Model file for the job. Use its own axes, mm. A direction names the side the tool comes from. Coordinates: 2 decimals unless noted, no trailing zeros. Write each loop counter-clockwise with the first axis right and the second up, starting at its lowest first coordinate (ties: lowest second). Pieces come first, ordered by that corner, then holes. Notation, with made-up numbers: M -29,-5.5 L 18,-5.5 A25 cw 18,21.5 Z; hole C 89.5,70 d10. An arc over 180 degrees is marked long. One line per question, with ' | ' between items. Start each with the question number.
(1) Wall check: probe 1 along X at (y, z) = (1.15, 15.5) (3 decimals); probe 2 along X at (y, z) = (0.9, -23.57) (3 decimals); probe 3 along Z at (x, y) = (15, 3.25) (1 decimal). Give the ranges that are in metal, low to high.
(2) Flat gauge pins, fed straight in: pin 1 Ø17.5 at (x, z) = (-14, 19.5) entering from -Y; pin 2 Ø4.5 at (x, z) = (-15.5, 15.5) entering from -Y; pin 3 Ø2 at (x, y) = (-20.5, -1.5) entering from -Z; pin 4 Ø8 at (x, z) = (5.5, 3) entering from -Y. Where does each tip first touch, or does it go through?
(3) Tool access for faces 1 (the face through (-18, 0, -21)), 2 (the face through (-18, 2, 12.5)), 3 (the face through (-28.625, 2, 19)): list every direction of +Z, -Z, +X, -X, +Y, -Y with a clear straight run to the whole face (end or side of a thin tool).
(4) Cut at D-D (y = -1.75). Write the cut outline in (x, z) (3 decimals).
(5) Two-plate mould, pull along X, no slides. Class faces 4 (the face through (-6.625, 2, 0)), 5 (the face through (0, 4, -13)), 6 (the face through (-1.1, -2.75, -0.4)), 7 (the face through (25.68, 1.97, -22.23)): +X half, -X half, draft (parallel to the pull), parting line (faces both ways), or undercut.
(6) Cut at B-B (y = 1.75). Count the separate pieces of the cut face and the enclosed holes in it, plus the area to 3 significant figures.
(7) Cut at C-C (z = 23.57). Write the cut outline in (x, y) (3 decimals).
(8) Cut at A-A (z = 15.5). Write the cut outline in (x, y) (3 decimals), plus the area to 3 significant figures.
from build123d import *

# Parameters (mm, degrees)
SKETCH1_R              = 2
SKETCH1_R_2            = 2.5
BOSS_EXTRUDE1_DEPTH    = 4
CUT_EXTRUDE2_DEPTH     = 23
CHAMFER2_SIZE          = 1
CUT_EXTRUDE3_START     = -4
CUT_EXTRUDE3_OUTLINE_W = 22
CUT_EXTRUDE3_OUTLINE_H = 25
CUT_EXTRUDE3_DEPTH     = 4
BOSS_EXTRUDE2_REACH    = 66.132


# Read off the part's stored shape, not the designer's step: Cut-Extrude3
with BuildPart() as part:
    # Sketch1 → Boss-Extrude1 (new body)
    with BuildSketch(Plane(origin=(0, 0, 0), x_dir=(1, 0, 0), z_dir=(0, 1, 0))):
        with BuildLine():
            Line((25.625, 28.625), (-25.625, 28.625))
            ThreePointArc((-25.625, 28.625), (-27.746320344, 27.746320344), (-28.625, 25.625))
            Line((-28.625, 25.625), (-28.625, -25.625))
            ThreePointArc((-28.625, -25.625), (-27.746320344, -27.746320344), (-25.625, -28.625))
            Line((-25.625, -28.625), (25.625, -28.625))
            ThreePointArc((25.625, -28.625), (27.746320344, -27.746320344), (28.625, -25.625))
            Line((28.625, -25.625), (28.625, 25.625))
            ThreePointArc((28.625, 25.625), (27.746320344, 27.746320344), (25.625, 28.625))
        make_face()
        with Locations(Location((-15.5, 15.5, 0), (0, 0, 270))):
            Circle(SKETCH1_R, mode=Mode.SUBTRACT)
        with Locations(Location((-23.57, 23.57, 0), (0, 0, 270))):
            Circle(SKETCH1_R_2, mode=Mode.SUBTRACT)
        with Locations(Location((23.57, 23.57, 0), (0, 0, 270))):
            Circle(SKETCH1_R_2, mode=Mode.SUBTRACT)
        with Locations(Location((15.5, 15.5, 0), (0, 0, 270))):
            Circle(SKETCH1_R, mode=Mode.SUBTRACT)
        with Locations(Location((15.5, -15.5, 0), (0, 0, 270))):
            Circle(SKETCH1_R, mode=Mode.SUBTRACT)
        with Locations(Location((-15.5, -15.5, 0), (0, 0, 270))):
            Circle(SKETCH1_R, mode=Mode.SUBTRACT)
        with Locations(Location((-23.57, -23.57, 0), (0, 0, 270))):
            Circle(SKETCH1_R_2, mode=Mode.SUBTRACT)
        with Locations(Location((23.57, -23.57, 0), (0, 0, 270))):
            Circle(SKETCH1_R_2, mode=Mode.SUBTRACT)
    extrude(amount=BOSS_EXTRUDE1_DEPTH)

    # Sketch3 → Cut-Extrude2 (cut)
    with BuildSketch(Plane.XY.offset(11.5)):
        Polygon((-28.125, 4), (-27.125, 3), (-26.125, 4), align=None)
        Polygon((-25.125, 4), (-24.125, 3), (-23.125, 4), align=None)
        Polygon((-22.125, 4), (-21.125, 3), (-20.125, 4), align=None)
        Polygon((-19.125, 4), (-18.125, 3), (-17.125, 4), align=None)
        Polygon((-16.125, 4), (-15.125, 3), (-14.125, 4), align=None)
        Polygon((-13.125, 4), (-12.125, 3), (-11.125, 4), align=None)
        Polygon((-10.125, 4), (-9.125, 3), (-8.125, 4), align=None)
        Polygon((-7.125, 4), (-6.125, 3), (-5.125, 4), align=None)
        Polygon((-4.125, 4), (-3.125, 3), (-2.125, 4), align=None)
        Polygon((-1.125, 4), (-0.125, 3), (0.875, 4), align=None)
        Polygon((1.875, 4), (2.875, 3), (3.875, 4), align=None)
        Polygon((4.875, 4), (5.875, 3), (6.875, 4), align=None)
        Polygon((7.875, 4), (8.875, 3), (9.875, 4), align=None)
        Polygon((10.875, 4), (11.875, 3), (12.875, 4), align=None)
        Polygon((13.875, 4), (14.875, 3), (15.875, 4), align=None)
        Polygon((16.875, 4), (17.875, 3), (18.875, 4), align=None)
        Polygon((19.875, 4), (20.875, 3), (21.875, 4), align=None)
        Polygon((22.875, 4), (23.875, 3), (24.875, 4), align=None)
        Polygon((25.875, 4), (26.875, 3), (27.875, 4), align=None)
    extrude(amount=-CUT_EXTRUDE2_DEPTH, mode=Mode.SUBTRACT)

    # Chamfer2
    chamfer2_edges = [part.edges().sort_by_distance(p)[0] for p in [
        (26.875, 4, -11.5),
        (23.875, 4, -11.5),
        (20.875, 4, -11.5),
        (17.875, 4, -11.5),
        (14.875, 4, -11.5),
        (11.875, 4, -11.5),
        (8.875, 4, -11.5),
        (5.875, 4, -11.5),
        (2.875, 4, -11.5),
        (-0.125, 4, -11.5),
        (-3.125, 4, -11.5),
        (-6.125, 4, -11.5),
        (-9.125, 4, -11.5),
        (-12.125, 4, -11.5),
        (-15.125, 4, -11.5),
        (-18.125, 4, -11.5),
        (-21.125, 4, -11.5),
        (-24.125, 4, -11.5),
        (-27.125, 4, -11.5),
        (26.875, 4, 11.5),
        (23.875, 4, 11.5),
        (20.875, 4, 11.5),
        (17.875, 4, 11.5),
        (14.875, 4, 11.5),
        (11.875, 4, 11.5),
        (8.875, 4, 11.5),
        (5.875, 4, 11.5),
        (2.875, 4, 11.5),
        (-0.125, 4, 11.5),
        (-3.125, 4, 11.5),
        (-6.125, 4, 11.5),
        (-9.125, 4, 11.5),
        (-12.125, 4, 11.5),
        (-15.125, 4, 11.5),
        (-18.125, 4, 11.5),
        (-21.125, 4, 11.5),
        (-24.125, 4, 11.5),
        (-27.125, 4, 11.5),
    ]]
    chamfer(chamfer2_edges, length=CHAMFER2_SIZE - 0.0001)  # a hair under: the kernel refuses the full size

    # Cut-Extrude3 outline → Cut-Extrude3 (cut)
    with BuildSketch(Plane.XZ.offset(CUT_EXTRUDE3_START)):
        with Locations((-17.625, 0)):
            Rectangle(CUT_EXTRUDE3_OUTLINE_W, CUT_EXTRUDE3_OUTLINE_H)
    extrude(amount=CUT_EXTRUDE3_DEPTH, mode=Mode.SUBTRACT)

    # Boss-Extrude2: up to this face of the body (flat: up to its plane)
    boss_extrude2_end = Plane(part.part.faces().sort_by_distance((0, 2, 28.625))[0])
    # Sketch5 → Boss-Extrude2 (add, up to the picked face)
    with BuildSketch(Plane(origin=(0, 0, -28.625), x_dir=(-1, 0, 0), z_dir=(0, 0, -1)), mode=Mode.PRIVATE) as boss_extrude2_sk1:
        with BuildLine():
            Line((6.625, 0), (-4.249281585, 0))
            ThreePointArc((-4.249281585, 0), (1.187859207, -2.75), (6.625, 0))
        make_face()
    boss_extrude2_tool1 = split(extrude(boss_extrude2_sk1.sketch, amount=-BOSS_EXTRUDE2_REACH, mode=Mode.PRIVATE), bisect_by=boss_extrude2_end, keep=Keep.BOTH, mode=Mode.PRIVATE)
    add(boss_extrude2_tool1.solids().sort_by(Axis((-1.187859, -1.121798, -28.625), (0, 0, 1)))[0])


solid = part.part
Filled in:
1) probe 1: -28.625 to -17.5, -13.5 to 13.5, 17.5 to 28.625 | probe 2: -28.625 to -26.07, -21.07 to 21.07, 26.07 to 28.625 | probe 3: -28.6 to -17.4, -13.6 to -11.7, 11.7 to 13.6, 17.4 to 28.6
2) pin 1: y = -1.39 | pin 2: y = 0 | pin 3: through | pin 4: y = -2.19
3) face 1: +Z, -Z, -X, -Y | face 2: -X, +Y, -Y | face 3: +Z, -Z, -X, +Y, -Y
4) outline: M -4.723,-28.625 L 2.348,-28.625 L 2.348,28.625 L -4.723,28.625 Z
5) face 4: -X half | face 5: draft | face 6: parting line | face 7: undercut
6) separate pieces: 1 | enclosed holes: 8 | area: 2,590 mm²
7) outline: M -28.625,0 L -26.07,0 L -26.07,4 L -28.625,4 Z; M -21.07,0 L -6.625,0 A6.75 ccw 4.249,0 L 21.07,0 L 21.07,4 L -21.07,4 Z; M 26.07,0 L 28.625,0 L 28.625,4 L 26.07,4 Z
8) outline: M -28.625,0 L -17.5,0 L -17.5,4 L -28.625,4 Z; M -13.5,0 L -6.625,0 A6.75 ccw 4.249,0 L 13.5,0 L 13.5,4 L -13.5,4 Z; M 17.5,0 L 28.625,0 L 28.625,4 L 17.5,4 Z | area: 218 mm²
